Geometry check sheet. Reference: the model listing, model coordinates, mm. Give positions to 0.01 mm unless a question says otherwise; leave off trailing zeros. Write each loop counter-clockwise with the first axis right and the second up, starting at its lowest first coordinate (ties: lowest second). Pieces come first, ordered by that corner, then holes. Notation, with made-up numbers: (60, 36) - (90, 36) arc R29 cw to (90, 73) - close; hole circle Ø2 at (18.25, 47). An arc over 180 degrees is marked (long way). Use a Markdown table: item, result.
```python
from build123d import *

# Parameters (mm, degrees)
F0_W = 14.2875
F0_H = 127
F2_T = -1.5875
F3_R = 2.54
F4_R = 0.79374


# Not quite as in the source:
# - a fillet or chamfer is up to 0.001 mm smaller than in the source, because OpenCascade refuses the exact size


with BuildPart() as f1:
    # F0 (on Front) → F1 (revolve)
    with BuildSketch(Plane.XZ):
        with Locations((7.14375, 0)):
            Rectangle(F0_W, F0_H)
    revolve(axis=Axis((0, 0, 0), (0, 0, -1)))

    # F2
    f2_openings = [f1.faces().sort_by_distance(p)[0] for p in [
        (0, 0, 63.5),
    ]]
    offset(amount=F2_T, openings=f2_openings)

    # F3
    f3_edges = [f1.edges().sort_by_distance(p)[0] for p in [
        (-14.2875, 0, -63.5),
    ]]
    fillet(f3_edges, radius=F3_R)

    # F4 (radius 0.79375 in the source; OpenCascade refuses exactly that, so slightly less here)
    f4_edges = [f1.edges().sort_by_distance(p)[0] for p in [
        (-14.2875, 0, 63.5),
        (-12.7, 0, 63.5),
    ]]
    fillet(f4_edges, radius=F4_R)


solid = f1.part
```
1) Section check B-B on z = -41.5. Record the boundary of the cut face in (x, y) (1 decimal).
Working result:
| item | result |
|---|---|
| outline | circle Ø28.6 at (0, 0); hole circle Ø25.4 at (0, 0) |
2) Depth check by flat-ended pin: P1, Ø3, axis at x = -10, z = 22, coming from the +Y side; P2, Ø2, axis at y = -2.5, z = 33, coming from the +X side; P3, Ø1, axis at x = 0, y = 9, coming from the +Z side. Enter the tip coordinate at first touch or a pass-through.
Working result:
| item | result |
|---|---|
| P1 | stops at y = 11.48 |
| P2 | stops at x = 14.21 |
| P3 | stops at z = -61.91 |
3) Material ranges on L1, parallel to X at y = 0, z = -14; L2, parallel to Z at x = 1, y = -2, recorded low to high. Write a range as from..to.
Working result:
| item | result |
|---|---|
| L1 | x = -14.29..-12.7, 12.7..14.29 |
| L2 | z = -63.5..-61.91 |
4) Mould release check, pull along X, two halves, no side actions. Record for faces 1 (the flat face through (0, 0, -63.5)), 2 (the flat face through (0, 0, -61.912)), 3 (the cylindrical face through (-14.274, -0.628, 1.739)): pulls with the +X half, pulls with the -X half, needs draft (parallel to the pull), parting line crosses it, or undercut.
Working result:
| item | result |
|---|---|
| face 1 | needs draft |
| face 2 | undercut |
| face 3 | parting line crosses it |
